Build history of the part. All positions in model axes, mm. A direction names the side the tool comes from. Round coordinates to 2 decimals unless told otherwise and drop trailing zeros. Loops run counter-clockwise (first coordinate to the right, second up) from the corner with the lowest first, then second, coordinate; pieces in that order, holes last. Notation, with made-up numbers: (41.5, 72.25) - (50.5, 72.25) arc R9 ccw to (50.5, 83.25) - close; hole circle Ø5 at (72.25, 67). An arc over 180 degrees is marked (long way). Use a Markdown table: item, result.
from build123d import *

# Parameters (mm, degrees)
PAD_DEPTH       = 40
POCKET_DEPTH    = 7.001
POCKET001_DEPTH = 7.001


with BuildPart() as part:
    # Sketch → Pad (new body)
    with BuildSketch(Plane.XZ):
        Polygon((-25, -16.524014), (25, -16.524014), (25, -9.524014), (15, -9.524014), (10, 13.475986), (5, 13.475986), (10.03446, 3.475986), (-9.96554, 3.475986), (-5, 13.475986), (-10, 13.475986), (-15, -9.524014), (-25, -9.524014), align=None)
    extrude(amount=PAD_DEPTH)

    # Sketch001 → Pocket (cut, through all)
    with BuildSketch(Plane(origin=(0, 0, -9.524014), x_dir=(-1, 0, 0), z_dir=(0, 0, 1))):
        with BuildLine():
            ThreePointArc((-17, 29), (-20, 32), (-23, 29))
            Line((-23, 29), (-23, 11))
            ThreePointArc((-23, 11), (-20, 8), (-17, 11))
            Line((-17, 29), (-17, 11))
        make_face()
    extrude(amount=-POCKET_DEPTH, mode=Mode.SUBTRACT)

    # Sketch002 → Pocket001 (cut, through all)
    with BuildSketch(Plane(origin=(0, 0, -9.524014), x_dir=(-1, 0, 0), z_dir=(0, 0, 1))):
        with BuildLine():
            ThreePointArc((23, 29), (20, 32), (17, 29))
            Line((17, 11), (17, 29))
            ThreePointArc((17, 11), (20, 8), (23, 11))
            Line((23, 29), (23, 11))
        make_face()
    extrude(amount=-POCKET001_DEPTH, mode=Mode.SUBTRACT)


solid = part.part
Q1. Which spindle directions (+Z, -Z, +X, -X, +Y, -Y) get a long thin tool onto all of the face, cutting with end or side? Do faces 1 (the face through (-16.6, -19.7, -9.524)), 2 (the face through (0, -20, 3.476)), 3 (the face through (-20, -8, -13)), 4 (the face through (23.4, -19.7, -9.524)). Say none if no direction does.
Results found:
| item | result |
|---|---|
| face 1 | +Z, -X, +Y, -Y |
| face 2 | +Y, -Y |
| face 3 | +Z, -Z |
| face 4 | +Z, +X, +Y, -Y |
Q2. Cut at B-B, the plane y = -16. List the corners of the cut face in (x, z), plus the area to 3 significant figures.
Results found:
| item | result |
|---|---|
| outline | (-25, -16.52) - (-23, -16.52) - (-23, -9.52) - (-25, -9.52) - close; (-17, -16.52) - (17, -16.52) - (17, -9.52) - (15, -9.52) - (10, 13.48) - (5, 13.48) - (10.03, 3.48) - (-9.97, 3.48) - (-5, 13.48) - (-10, 13.48) - (-15, -9.52) - (-17, -9.52) - close; (23, -16.52) - (25, -16.52) - (25, -9.52) - (23, -9.52) - close |
| area | 691 mm2 |
Q3. Cut at C-C, the plane z = 6.5. List the corners of the cut face in (x, y), plus the area to 3 significant figures.
Results found:
| item | result |
|---|---|
| outline | (-11.52, -40) - (-8.46, -40) - (-8.46, 0) - (-11.52, 0) - close; (8.51, -40) - (11.52, -40) - (11.52, 0) - (8.51, 0) - close |
| area | 242 mm2 |
Q4. Pull direction X, two halves, no side cores. Call faces 5 (the face through (0, 0, -5)), 6 (the face through (12.535, -19.72, 1.815)), 7 (the face through (-17, -20, -13)): pulls with the +X half, pulls with the -X half, needs draft (parallel to the pull), parting line crosses it, or undercut.
Results found:
| item | result |
|---|---|
| face 5 | needs draft |
| face 6 | pulls with the +X half |
| face 7 | undercut |
Q5. Drop flat-ended pins along their axis: pin 1 (1 mm diameter, centred on y = -17, z = 8.5, fed in from -X); pin 2 (10 mm diameter, centred on x = -16, z = 3.5, fed in from -Y); pin 3 (5 mm diameter, centred on x = -18.5, y = -14.5, fed in from +Z); pin 4 (8 mm diameter, centred on y = -27, z = 3, fed in from -X). Give the stop position or say it passes through.
Results found:
| item | result |
|---|---|
| pin 1 | stops at x = -11.19 |
| pin 2 | stops at y = -40 |
| pin 3 | stops at z = -9.52 |
| pin 4 | stops at x = -13.15 |
Q6. Cut at A-A, the plane x = -20. List the corners of the cut face in (y, z).
Results found:
| item | result |
|---|---|
| outline | (-40, -16.52) - (-32, -16.52) - (-32, -9.52) - (-40, -9.52) - close; (-8, -16.52) - (0, -16.52) - (0, -9.52) - (-8, -9.52) - close |
Q7. Probe line 1 (X direction, y = -21, z = -12); line 2 (X direction, y = -28, z = 11.25); line 3 (Z direction, x = 2, y = -30.5). List the from-to ranges inside material, lowest first.
Results found:
| item | result |
|---|---|
| line 1 | x = -25 to -23, -17 to 17, 23 to 25 |
| line 2 | x = -10.48 to -6.11, 6.12 to 10.48 |
| line 3 | z = -16.52 to 3.48 |
Q8. Cut at D-D, the plane y = -33. List the corners of the cut face in (x, z).
Results found:
| item | result |
|---|---|
| outline | (-25, -16.52) - (25, -16.52) - (25, -9.52) - (15, -9.52) - (10, 13.48) - (5, 13.48) - (10.03, 3.48) - (-9.97, 3.48) - (-5, 13.48) - (-10, 13.48) - (-15, -9.52) - (-25, -9.52) - close |
